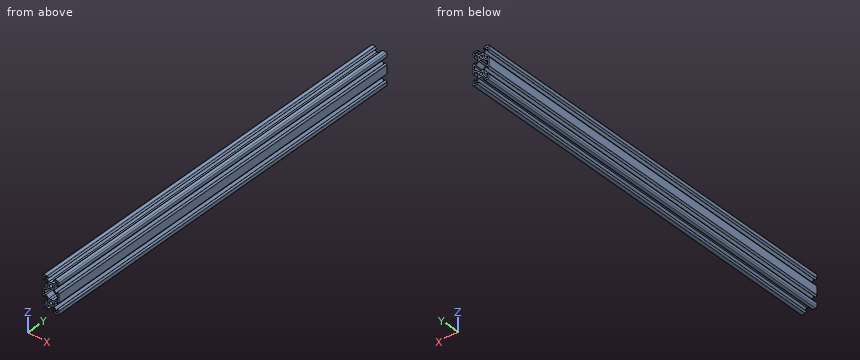
from build123d import *

# Parameters (mm, degrees)
F2_DEPTH = 480


with BuildPart() as f2:
    # F0 (on Front) → F2 (new body)
    with BuildSketch(Plane.XZ):
        with BuildLine():
            Line((5.0927712857, 0), (1.5, 0))
            ThreePointArc((1.5, 0), (0.4393398282, -0.4393398282), (0, -1.5))
            Line((0, -1.5), (0, -5.0927712857))
            ThreePointArc((0, -5.0927712857), (0.0601351693, -5.3950911973), (0.2313856429, -5.6513856429))
            Line((0.2313856429, -5.6513856429), (1.69, -7.11))
            Line((1.69, -7.11), (1.8, -7.11))
            Line((1.8, -7.11), (1.8, -4.5006601718))
            Line((1.8, -4.5006601718), (3.44, -4.5006601718))
            Line((3.44, -4.5006601718), (6.1000000155, -7.1606601718))
            Line((6.1000000155, -7.1606601718), (6.1000000155, -9.9))
            Line((6.1000000155, -9.9), (6.2000000155, -10))
            Line((6.2000000155, -10), (6.1000000155, -10.1))
            Line((6.1000000155, -10.1), (6.1000000155, -12.8393398605))
            Line((6.1000000155, -12.8393398605), (3.44, -15.4993398916))
            Line((3.44, -15.4993398916), (1.8, -15.4993398916))
            Line((1.8, -15.4993398916), (1.8, -12.8893398916))
            Line((1.8, -12.8893398916), (1.69, -12.8893398916))
            Line((1.69, -12.8893398916), (0.2313856429, -14.3479542487))
            ThreePointArc((0.2313856429, -14.3479542487), (0.0601351693, -14.6042486943), (0, -14.9065686059))
            Line((0, -14.9065686059), (0, -20))
            Line((0, -20), (0, -25.0934313941))
            ThreePointArc((0, -25.0934313941), (0.0601351693, -25.3957513057), (0.2313856429, -25.6520457513))
            Line((0.2313856429, -25.6520457513), (1.69, -27.1106601084))
            Line((1.69, -27.1106601084), (1.8, -27.1106601084))
            Line((1.8, -27.1106601084), (1.8, -24.5006601084))
            Line((1.8, -24.5006601084), (3.44, -24.5006601084))
            Line((3.44, -24.5006601084), (6.1000000155, -27.1606601395))
            Line((6.1000000155, -27.1606601395), (6.1000000155, -29.9))
            Line((6.1000000155, -29.9), (6.2000000155, -30))
            Line((6.2000000155, -30), (6.1000000155, -30.1))
            Line((6.1000000155, -30.1), (6.1000000155, -32.8393398282))
            Line((6.1000000155, -32.8393398282), (3.44, -35.4993398282))
            Line((3.44, -35.4993398282), (1.8, -35.4993398282))
            Line((1.8, -35.4993398282), (1.8, -32.89))
            Line((1.8, -32.89), (1.69, -32.89))
            Line((1.69, -32.89), (0.2313856429, -34.3486143571))
            ThreePointArc((0.2313856429, -34.3486143571), (0.0601351693, -34.6049088027), (0, -34.9072287143))
            Line((0, -34.9072287143), (0, -38.5))
            ThreePointArc((0, -38.5), (0.4393398282, -39.5606601718), (1.5, -40))
            Line((1.5, -40), (5.0927712857, -40))
            ThreePointArc((5.0927712857, -40), (5.3950911973, -39.9398648307), (5.6513856429, -39.7686143571))
            Line((5.6513856429, -39.7686143571), (7.11, -38.31))
            Line((7.11, -38.31), (7.11, -38.2))
            Line((7.11, -38.2), (4.5006601718, -38.2))
            Line((4.5006601718, -38.2), (4.5006601718, -36.56))
            Line((4.5006601718, -36.56), (7.1606601873, -33.9))
            Line((7.1606601873, -33.9), (9.9000000155, -33.9))
            Line((9.9000000155, -33.9), (10.0000000478, -33.8000000323))
            Line((10.0000000478, -33.8000000323), (10.1000000802, -33.9))
            Line((10.1000000802, -33.9), (12.8393399084, -33.9))
            Line((12.8393399084, -33.9), (15.4993399239, -36.56))
            Line((15.4993399239, -36.56), (15.4993399239, -38.2))
            Line((15.4993399239, -38.2), (12.8900000957, -38.2))
            Line((12.8900000957, -38.2), (12.8900000957, -38.31))
            Line((12.8900000957, -38.31), (14.3486144528, -39.7686143571))
            ThreePointArc((14.3486144528, -39.7686143571), (14.6049088984, -39.9398648307), (14.90722881, -40))
            Line((14.90722881, -40), (18.5000000957, -40))
            ThreePointArc((18.5000000957, -40), (19.5606602675, -39.5606601718), (20.0000000957, -38.5))
            Line((20.0000000957, -38.5), (20.0000000957, -34.9072287143))
            ThreePointArc((20.0000000957, -34.9072287143), (19.9398649264, -34.6049088027), (19.7686144528, -34.3486143571))
            Line((19.7686144528, -34.3486143571), (18.3100000957, -32.89))
            Line((18.3100000957, -32.89), (18.2000000957, -32.89))
            Line((18.2000000957, -32.89), (18.2000000957, -35.4993398282))
            Line((18.2000000957, -35.4993398282), (16.5600000957, -35.4993398282))
            Line((16.5600000957, -35.4993398282), (13.9000000802, -32.8393398282))
            Line((13.9000000802, -32.8393398282), (13.9000000802, -30.1))
            Line((13.9000000802, -30.1), (13.8000000802, -30))
            Line((13.8000000802, -30), (13.9000000802, -29.9))
            Line((13.9000000802, -29.9), (13.9000000802, -27.1606601395))
            Line((13.9000000802, -27.1606601395), (16.5600000957, -24.5006601084))
            Line((16.5600000957, -24.5006601084), (18.2000000957, -24.5006601084))
            Line((18.2000000957, -24.5006601084), (18.2000000957, -27.1106601084))
            Line((18.2000000957, -27.1106601084), (18.3100000957, -27.1106601084))
            Line((18.3100000957, -27.1106601084), (19.7686144528, -25.6520457513))
            ThreePointArc((19.7686144528, -25.6520457513), (19.9398649264, -25.3957513057), (20.0000000957, -25.0934313941))
            Line((20.0000000957, -25.0934313941), (20.0000000957, -20))
            Line((20.0000000957, -20), (20.0000000957, -14.9065686059))
            ThreePointArc((20.0000000957, -14.9065686059), (19.9398649264, -14.6042486943), (19.7686144528, -14.3479542487))
            Line((19.7686144528, -14.3479542487), (18.3100000957, -12.8893398916))
            Line((18.3100000957, -12.8893398916), (18.2000000957, -12.8893398916))
            Line((18.2000000957, -12.8893398916), (18.2000000957, -15.4993398916))
            Line((18.2000000957, -15.4993398916), (16.5600000957, -15.4993398916))
            Line((16.5600000957, -15.4993398916), (13.9000000802, -12.8393398605))
            Line((13.9000000802, -12.8393398605), (13.9000000802, -10.1))
            Line((13.9000000802, -10.1), (13.8000000802, -10))
            Line((13.8000000802, -10), (13.9000000802, -9.9))
            Line((13.9000000802, -9.9), (13.9000000802, -7.1606601718))
            Line((13.9000000802, -7.1606601718), (16.5600000957, -4.5006601718))
            Line((16.5600000957, -4.5006601718), (18.2000000957, -4.5006601718))
            Line((18.2000000957, -4.5006601718), (18.2000000957, -7.11))
            Line((18.2000000957, -7.11), (18.3100000957, -7.11))
            Line((18.3100000957, -7.11), (19.7686144528, -5.6513856429))
            ThreePointArc((19.7686144528, -5.6513856429), (19.9398649264, -5.3950911973), (20.0000000957, -5.0927712857))
            Line((20.0000000957, -5.0927712857), (20.0000000957, -1.5))
            ThreePointArc((20.0000000957, -1.5), (19.5606602675, -0.4393398282), (18.5000000957, 0))
            Line((18.5000000957, 0), (14.90722881, 0))
            ThreePointArc((14.90722881, 0), (14.6049088984, -0.0601351693), (14.3486144528, -0.2313856429))
            Line((14.3486144528, -0.2313856429), (12.8900000957, -1.69))
            Line((12.8900000957, -1.69), (12.8900000957, -1.8))
            Line((12.8900000957, -1.8), (15.4993399239, -1.8))
            Line((15.4993399239, -1.8), (15.4993399239, -3.44))
            Line((15.4993399239, -3.44), (12.8393399084, -6.1))
            Line((12.8393399084, -6.1), (10.1000000802, -6.1))
            Line((10.1000000802, -6.1), (10.0000000478, -6.1999999677))
            Line((10.0000000478, -6.1999999677), (9.9000000155, -6.1))
            Line((9.9000000155, -6.1), (7.1606601873, -6.1))
            Line((7.1606601873, -6.1), (4.5006601718, -3.44))
            Line((4.5006601718, -3.44), (4.5006601718, -1.8))
            Line((4.5006601718, -1.8), (7.11, -1.8))
            Line((7.11, -1.8), (7.11, -1.69))
            Line((7.11, -1.69), (5.6513856429, -0.2313856429))
            ThreePointArc((5.6513856429, -0.2313856429), (5.3950911973, -0.0601351693), (5.0927712857, 0))
        make_face()
        Polygon((1.8, -38.2), (1.8, -36.57), (2.34, -36.57), (3.43, -37.66), (3.43, -38.2), align=None, mode=Mode.SUBTRACT)
        with BuildLine():
            ThreePointArc((10.0000000478, -27.9), (11.4849242883, -28.5150757595), (12.1000000478, -30))
            ThreePointArc((12.1000000478, -30), (11.4849242883, -31.4849242405), (10.0000000478, -32.1))
            ThreePointArc((10.0000000478, -32.1), (8.5150758074, -31.4849242405), (7.9000000478, -30))
            ThreePointArc((7.9000000478, -30), (8.5150758074, -28.5150757595), (10.0000000478, -27.9))
        make_face(mode=Mode.SUBTRACT)
        Polygon((17.6600000957, -36.57), (18.2000000957, -36.57), (18.2000000957, -38.2), (16.5700000957, -38.2), (16.5700000957, -37.66), align=None, mode=Mode.SUBTRACT)
        Polygon((9.9000000478, -13.9000000323), (10.0000000478, -13.8000000323), (10.1000000478, -13.9000000323), (12.8393399084, -13.9000000323), (16.2400000478, -17.3006601916), (18.2000000478, -17.3006601916), (18.2000000478, -20), (18.2000000478, -22.6993398084), (16.2400000478, -22.6993398084), (12.8393399084, -26.0999999677), (10.1000000478, -26.0999999677), (10.0000000478, -26.1999999677), (9.9000000478, -26.0999999677), (7.1606601873, -26.0999999677), (3.7600000478, -22.6993398084), (1.8000000478, -22.6993398084), (1.8000000478, -20), (1.8000000478, -17.3006601916), (3.7600000478, -17.3006601916), (7.1606601873, -13.9000000323), align=None, mode=Mode.SUBTRACT)
        Polygon((1.8, -3.43), (1.8, -1.8), (3.43, -1.8), (3.43, -2.34), (2.34, -3.43), align=None, mode=Mode.SUBTRACT)
        with BuildLine():
            ThreePointArc((7.9000000478, -10), (8.5150758074, -8.5150757595), (10.0000000478, -7.9))
            ThreePointArc((10.0000000478, -7.9), (11.4849242883, -8.5150757595), (12.1000000478, -10))
            ThreePointArc((12.1000000478, -10), (11.4849242883, -11.4849242405), (10.0000000478, -12.1))
            ThreePointArc((10.0000000478, -12.1), (8.5150758074, -11.4849242405), (7.9000000478, -10))
        make_face(mode=Mode.SUBTRACT)
        Polygon((16.5700000957, -2.34), (16.5700000957, -1.8), (18.2000000957, -1.8), (18.2000000957, -3.43), (17.6600000957, -3.43), align=None, mode=Mode.SUBTRACT)
    extrude(amount=F2_DEPTH)


solid = f2.part
Could you check a few things on this model? Use its own coordinates, in mm. Coordinates: 2 decimals unless noted, no trailing zeros. Put each result on its own line as item: value. Start each with the question number.
Q1. Please list where these lines run through material, in increasing order: L1, parallel to Z at x = 3.5, y = -357; L2, parallel to Z at x = 9, y = -171.5; L3, parallel to X at y = -212.5, z = -34.
Q2. I want a section at A-A on y = -73. Count the separate pieces of the cut face and the enclosed holes in it, plus the area to 3 significant figures.
Q3. I'm going to push flat-ended pins straight in: P1, Ø1, axis at x = 10, y = -366, coming from the -Z side; P2, Ø3, axis at y = -271, z = -33, coming from the -X side; P3, Ø0.8, axis at x = 9, y = -175, coming from the +Z side. Where does each tip first touch, or does it pass through?
Checks:
1. L1: -40 to -35.44, -24.56 to -22.7, -17.3 to -15.44, -4.56 to 0
1. L2: -33.9 to -31.85, -28.15 to -26.1, -13.9 to -11.85, -8.15 to -6.1
1. L3: 0.58 to 1.8, 4.94 to 7.06, 12.94 to 15.06, 18.2 to 19.42
2. separate pieces: 1
2. enclosed holes: 7
2. area: 291 mm²
3. P1: z = -33.9
3. P2: x = 0.11
3. P3: z = -6.1
